Verification items for the finished model (mm, model axes). Face numbers are marked on the shaded views. Give positions to 0.01 mm unless a question says otherwise; leave off trailing zeros. Order: outer loops, then holes, each group sorted by start corner. A loop starts at its lowest first (then second) coordinate and runs counter-clockwise, first axis right, second up. Notation, with made-up numbers: (-29.75, 41) -> (-13.75, 41) arc R20 cw to (-13.75, 49) -> close; hole circle Ø1 at (-34, 10.25). An arc over 180 degrees is marked (long way). Return JSON: item names as keys, results as strings. Group by question number.
(1) Thickness scan on line 1 along X through (y, z) = (106.5, -173); line 2 along X through (y, z) = (57, -326.5); line 3 along Z through (x, y) = (995, 86). Record the ranges inside material, lowest first.
(2) Depth check by flat-ended pin: pin 1 Ø6 at (y, z) = (95.5, -391.5) entering from -X; pin 2 Ø4 at (y, z) = (20, -417.5) entering from -X; pin 3 Ø8 at (y, z) = (100, -568.5) entering from +X. Enter the tip coordinate at first touch or a pass-through.
(3) Cross-section at C-C on y = 62. Enter the section's corners in (x, z).
(4) Cross-section at A-A on x = 1934. Enter the section's corners in (y, z).
(5) Cross-section at B-B on z = -51. Enter the section's corners in (x, y), then the cut area to 3 significant figures.
(6) Release check for a two-part mould opening along X. For the marked faces 1 and 2 record: pulls with the +X half, pulls with the -X half, needs draft (parallel to the pull), parting line crosses it, or undercut.
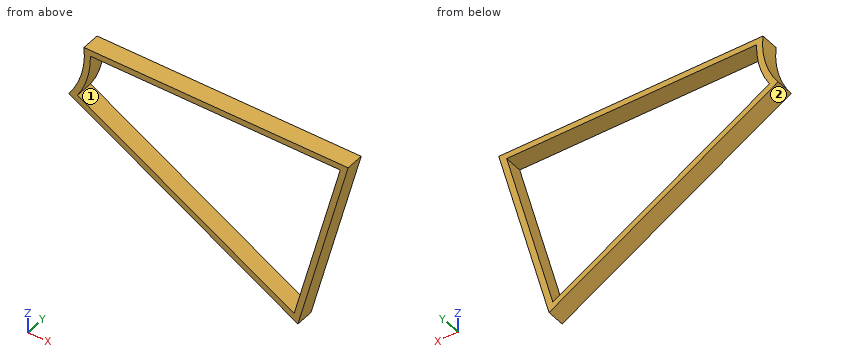
Autodesk Inventor part; units mm, degrees
ref_plane "YZ Plane" through (0, 0, 0) normal (1, 0, 0) x (0, 1, 0)
ref_plane "XZ Plane" through (0, 0, 0) normal (0, 1, 0) x (-1, 0, 0)
ref_plane "XY Plane" through (0, 0, 0) normal (0, 0, 1) x (1, 0, 0)
sketch "Sketch1" plane through (0, 0, 0) normal (0, 1, 0) x (-1, 0, 0)
  line L0 (0, 0) -> (-3000, 0) construction
  line L1 (0, 0) -> (-2598.0762, -1500) construction
  line L2 (0, 0) -> (3000, 0) construction
  arc A0 (-497.4937, 50) -> (-402.0602, -297.2332) centre (0, 0) ccw
  line L3 (-497.4937, 50) -> (-2157.4937, 50)
  line L4 (-2157.4937, 50) -> (-1841.7345, -1128.4295)
  line L5 (-2157.4937, 50) -> (-937.4937, 50) construction
  line L6 (-1841.7345, -1128.4295) -> (1158.2655, -1128.4295) construction
  line L7 (-1841.7345, -1128.4295) -> (-402.0602, -297.2332)
  arc A1 (-537.8662, 12) -> (-456.459, -284.7617) centre (0, 0) ccw
  line L8 (-2107.9712, 12) -> (-537.8662, 12)
  line L9 (-456.459, -284.7617) -> (-1817.8467, -1070.7593)
  line L10 (-2107.9712, 12) -> (-1817.8467, -1070.7593)
  dimension "d1" = 3000
  dimension "d2" = 150
  dimension "d3" = 1000
  dimension "d11" = 50
  dimension "d12" = 1660
  dimension "d13" = 1220
  dimension "d14" = 75
extrude "Extrusion2" add sketch "Sketch1" along normal blind 114
properties part number "panelAflat" material "Wood (Birch)"
Verdict:
{
 "1": {"line 1": "469.12 to 509.43, 2058.4 to 2097.74", "line 2": "452.75 to 528.75, 2017.27 to 2056.61", "line 3": "-639.57 to -595.69, 12 to 50"},
 "2": {"pin 1": "x = 560.14", "pin 2": "x = 606.9", "pin 3": "x = 1992.84"},
 "3": {"outline": "(402.06, -297.23) -> (1841.73, -1128.43) -> (2157.49, 50) -> (497.49, 50) arc R500 cw to start; hole (456.46, -284.76) -> (1817.85, -1070.76) -> (2107.97, 12) -> (537.87, 12) arc R538 cw to start"},
 "4": {"outline": "(0, -784.09) -> (114, -784.09) -> (114, -637.27) -> (0, -637.27) -> close; (0, 12) -> (114, 12) -> (114, 50) -> (0, 50) -> close"},
 "5": {"outline": "(497.39, 0) -> (535.58, 0) -> (535.58, 114) -> (497.39, 114) -> close; (2091.09, 0) -> (2130.43, 0) -> (2130.43, 114) -> (2091.09, 114) -> close", "area": "8,840 mm²"},
 "6": {"face 1": "undercut", "face 2": "pulls with the -X half"}
}
